from build123d import *

# Parameters (mm, degrees)
SKETCH1_W           = 11
SKETCH1_H           = 25
BOSS_EXTRUDE1_DEPTH = 9
SKETCH2_W           = 11
SKETCH2_H           = 3
SKETCH2_H_2         = 3.765669969
CUT_EXTRUDE2_DEPTH  = 29.757607689
CUT_EXTRUDE3_DEPTH  = 17.65
BOSS_EXTRUDE2_START = -6.96567
SKETCH4_R           = 1
BOSS_EXTRUDE2_DEPTH = 6.86567
SKETCH5_R           = 2
SKETCH5_R_2         = 1
BOSS_EXTRUDE3_DEPTH = 1
SKETCH6_R           = 1
BOSS_EXTRUDE4_DEPTH = 10


with BuildPart() as part:
    # Sketch1 → Boss-Extrude1 (new body)
    with BuildSketch(Plane(origin=(0, 0, 0), x_dir=(1, 0, 0), z_dir=(0, 1, 0))):
        with Locations((5.5, 12.5)):
            Rectangle(SKETCH1_W, SKETCH1_H)
    extrude(amount=BOSS_EXTRUDE1_DEPTH)

    # Sketch2 → Cut-Extrude2 (cut, through all)
    with BuildSketch(Plane(origin=(0, 9, 0), x_dir=(1, 0, 0), z_dir=(0, 1, 0))):
        with Locations((5.5, 19.534330031)):
            Rectangle(SKETCH2_W, SKETCH2_H)
        with Locations((5.5, 23.017165016)):
            Rectangle(SKETCH2_W, SKETCH2_H_2)
    extrude(amount=-CUT_EXTRUDE2_DEPTH, mode=Mode.SUBTRACT)


with BuildPart() as cut_extrude2_piece_1:
    # of the separate pieces the step leaves, piece 1, a body of its own (cut_extrude2_pieces)
    add(part.part.solids().sort_by_distance((0, 0, 0))[0])

    # Sketch3 → Cut-Extrude3 (cut)
    with BuildSketch(Plane.XY):
        with BuildLine():
            Line((11, 9), (10.03742995, 9))
            ThreePointArc((10.03742995, 9), (10.756666057, 6.800898811), (11, 4.500000028))
            Line((11, 4.500000028), (11, 9))
        make_face()
        with BuildLine():
            Line((11, 0), (11, 4.500000028))
            ThreePointArc((11, 4.500000028), (10.756666063, 2.199101216), (10.03742995, 0))
            Line((10.03742995, 0), (11, 0))
        make_face()
        with BuildLine():
            ThreePointArc((0.96257005, 0), (0.243333935, 2.199101225), (0, 4.500000045))
            Line((0, 4.500000045), (0, 0))
            Line((0, 0), (0.96257005, 0))
        make_face()
        with BuildLine():
            ThreePointArc((0, 4.500000045), (0.243333945, 6.800898819), (0.96257005, 9))
            Line((0.96257005, 9), (0, 9))
            Line((0, 9), (0, 4.500000045))
        make_face()
    extrude(amount=-CUT_EXTRUDE3_DEPTH, mode=Mode.SUBTRACT)



with BuildPart() as cut_extrude2_piece_2:
    # of the separate pieces the step leaves, piece 2, a body of its own (cut_extrude2_pieces)
    add(part.part.solids().sort_by_distance((0, 0, -21.134330031))[0])


with BuildPart() as cut_extrude2_piece_3:
    # of the separate pieces the step leaves, piece 3, a body of its own (cut_extrude2_pieces)
    add(part.part.solids().sort_by_distance((0, 0, -25))[0])


with BuildPart() as cut_extrude2_piece_1_1:
    add(cut_extrude2_piece_1.part)

    add(cut_extrude2_piece_2.part)  # Boss-Extrude2 merges Cut-Extrude2 piece 2

    add(cut_extrude2_piece_3.part)  # Boss-Extrude2 merges Cut-Extrude2 piece 3
    # Sketch4 → Boss-Extrude2 (add)
    with BuildSketch(Plane(origin=(0, 0, -25), x_dir=(-1, 0, 0), z_dir=(0, 0, -1)).offset(BOSS_EXTRUDE2_START)):
        with Locations((-2, 7)):
            Circle(SKETCH4_R)
        with Locations(Location((-9, 2, 0), (0, 0, 180))):
            Circle(SKETCH4_R)
    extrude(amount=BOSS_EXTRUDE2_DEPTH)

    # Sketch5 → Boss-Extrude3 (add)
    with BuildSketch(Plane.XY):
        with Locations(Location((5.5, 4.5, 0), (0, 0, 180))):
            Circle(SKETCH5_R)
        with Locations((5.5, 4.5)):
            Circle(SKETCH5_R_2, mode=Mode.SUBTRACT)
    extrude(amount=BOSS_EXTRUDE3_DEPTH)

    # Sketch6 → Boss-Extrude4 (add)
    with BuildSketch(Plane(origin=(0, 0, -25), x_dir=(-1, 0, 0), z_dir=(0, 0, -1))):
        with Locations(Location((-5.5, 4.5, 0), (0, 0, 180))):
            Circle(SKETCH6_R)
    extrude(amount=BOSS_EXTRUDE4_DEPTH)


solid = cut_extrude2_piece_1_1.part
The listing builds one solid part. Answer for the finished solid, in the listing's coordinates (mm). A direction names the side the tool comes from. Round coordinates to 2 decimals unless told otherwise and drop trailing zeros. Write each loop counter-clockwise with the first axis right and the second up, starting at its lowest first coordinate (ties: lowest second). Pieces come first, ordered by that corner, then holes. Notation, with made-up numbers: (18, -29) - (32, -29) arc R23 cw to (32, -8) - close; hole circle Ø3 at (4, -38). An arc over 180 degrees is marked (long way). Use a Markdown table: item, result. Add a question column.
1. The part is cut by section D-D (z = -10). Write down the section's boundary in (x, y).
2. Flat-ended cylindrical pins translate along their axes: P1, Ø0.5, axis at x = 0.5, y = 6, coming from the +Z side; P2, Ø3, axis at y = 7.5, z = -28, coming from the +X side. Find the tip coordinate at first contact, or state that the pin passes through.
3. For a pull along X with two mould halves and no side action, classify faces 4 (the face through (4.763, 5.176, 0.493)), 5 (the face through (0.3, 7.9, -17.65)), 6 (the face through (4.763, 3.824, -29.93)) as +X half, -X half, draft (parallel to the pull), parting line (faces both ways), or undercut.
4. The part is cut by section B-B (y = 0.5). Write down the section's boundary in (x, z), and give its area (3 significant figures).
5. Consider line 1 (Y direction, x = 5.5, z = 0.6); line 2 (X direction, y = 6.75, z = -21.5); line 3 (X direction, y = 7.5, z = -23.5). Determine where each line is inside the solid, lowest interval first.
6. The part is cut by section C-C (z = -21.5). Write down the section's boundary in (x, y), and give its area (3 significant figures).
7. A tool of negligible diameter and unlimited length cuts with its end or side. For faces 1 (the face through (5, 4, 0)), 2 (the face through (0.3, 1.1, -17.65)), 3 (the face through (8.2, 2.6, -23)), from which of +Z, -Z, +X, -X, +Y, -Y can it reach the whole face along a straight path? Write none if from no direction.
8. The part is cut by section A-A (x = 5.5). Write down the section's boundary in (y, z).
Reported:
| question | item | result |
|---|---|---|
| 1 | outline | (0.96, 0) - (10.04, 0) arc R11 ccw to (10.04, 9) - (0.96, 9) arc R11 ccw to start |
| 2 | P1 | z = 0 |
| 2 | P2 | through |
| 3 | face 4 | undercut |
| 3 | face 5 | draft |
| 3 | face 6 | parting line |
| 4 | outline | (0, -25) - (11, -25) - (11, -24.9) - (0, -24.9) - close; (0, -21.13) - (11, -21.13) - (11, -21.03) - (0, -21.03) - close; (0, -18.03) - (11, -18.03) - (11, -17.65) - (10.25, -17.65) - (10.25, 0) - (0.75, 0) - (0.75, -17.65) - (0, -17.65) - close |
| 4 | area | 174 mm^2 |
| 5 | line 1 | 2.5 to 3.5, 5.5 to 6.5 |
| 5 | line 2 | 1.03 to 2.97 |
| 5 | line 3 | 1.13 to 2.87 |
| 6 | outline | circle Ø2 at (2, 7); circle Ø2 at (9, 2) |
| 6 | area | 6.28 mm^2 |
| 7 | face 1 | +Z |
| 7 | face 2 | +Z, -X, -Y |
| 7 | face 3 | none |
| 8 | outline | (0, -25) - (3.5, -25) - (3.5, -35) - (5.5, -35) - (5.5, -25) - (9, -25) - (9, -24.9) - (0, -24.9) - close; (0, -21.13) - (9, -21.13) - (9, -21.03) - (0, -21.03) - close; (0, -18.03) - (9, -18.03) - (9, 0) - (6.5, 0) - (6.5, 1) - (5.5, 1) - (5.5, 0) - (3.5, 0) - (3.5, 1) - (2.5, 1) - (2.5, 0) - (0, 0) - close |
